The listing builds one solid part. Answer for the finished solid, in the listing's coordinates (mm). Face numbers are marked on the shaded views. A direction names the side the tool comes from. Give positions to 0.01 mm unless a question says otherwise; leave off trailing zeros. Write each loop counter-clockwise with the first axis right and the second up, starting at its lowest first coordinate (ties: lowest second). Pieces come first, ordered by that corner, then holes. Notation, with made-up numbers: (61.5, -7) -> (77.5, -7) arc R13 ccw to (77.5, 11) -> close; hole circle Ø10 at (14, 71). An arc over 180 degrees is marked (long way). Put each result on its own line as item: value. Start each with the question number.
1) Find the intervals of material crossed by line 1 along X through (y, z) = (-6.25, 0); line 2 along Y through (x, z) = (2.5, -3); line 3 along X through (y, z) = (-4, 0), in increasing order. Write a range as from..to.
2) Flat-ended cylindrical pins translate along their axes: pin 1 Ø10 at (y, z) = (1.5, -15.5) entering from -X; pin 2 Ø2 at (x, z) = (0, 12.5) entering from +Y; pin 3 Ø12 at (y, z) = (-61.5, 10) entering from +X. Find the tip coordinate at first contact, or state that the pin passes through.
3) For the marked faces 1, 2 and 3, determine the directions among +Z, -Z, +X, -X, +Y, -Y from which every point of the face is accessible in a straight line to the end or side of a thin tool.
4) A cutting plane is placed at B-B (y = -66). Write down the section's boundary in (x, z).
5) A cutting plane is placed at C-C (y = -46). Write down the section's boundary in (x, z), then the cut area to 3 significant figures.
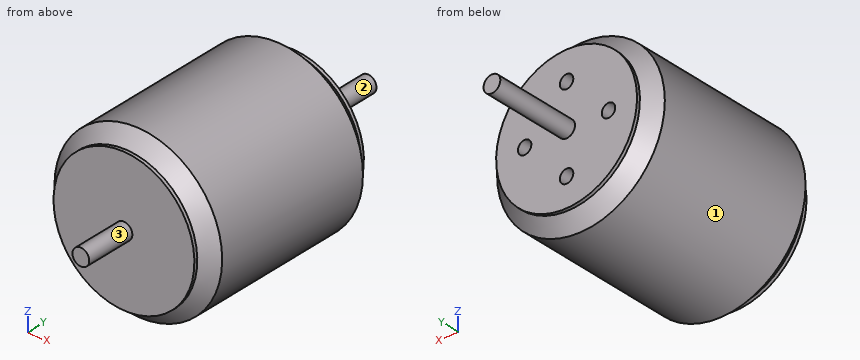
from build123d import *

# Parameters (mm, degrees)
SKETCH1_R           = 21
BOSS_EXTRUDE1_DEPTH = 59
SKETCH1_3_R         = 2.5
BOSS_EXTRUDE2_DEPTH = 26
SKETCH1_4_R         = 2
CUT_EXTRUDE1_DEPTH  = 10
BOSS_EXTRUDE3_START = -5
SKETCH1_5_R         = 25
SKETCH1_5_R_2       = 21
BOSS_EXTRUDE3_DEPTH = 49
CHAMFER1_SIZE       = 4
BOSS_EXTRUDE4_START = -74
SKETCH1_6_R         = 2.5
BOSS_EXTRUDE4_DEPTH = 15


with BuildPart() as part:
    # Sketch1 → Boss-Extrude1 (new body)
    with BuildSketch(Plane(origin=(0, 0, 0), x_dir=(1, 0, 0), z_dir=(0, 1, 0))):
        with Locations(Location((0, 0, 0), (0, 0, 270))):
            Circle(SKETCH1_R)
    extrude(amount=-BOSS_EXTRUDE1_DEPTH)

    # Sketch1<3> → Boss-Extrude2 (add)
    with BuildSketch(Plane(origin=(0, 0, 0), x_dir=(1, 0, 0), z_dir=(0, 1, 0))):
        with Locations(Location((0, 0, 0), (0, 0, 90))):
            Circle(SKETCH1_3_R)
    extrude(amount=BOSS_EXTRUDE2_DEPTH)

    # Sketch1<4> → Cut-Extrude1 (cut)
    with BuildSketch(Plane(origin=(0, 0, 0), x_dir=(1, 0, 0), z_dir=(0, 1, 0))):
        with Locations(Location((-12.5, 0, 0), (0, 0, 270))):
            Circle(SKETCH1_4_R)
        with Locations(Location((0, 12.5, 0), (0, 0, 270))):
            Circle(SKETCH1_4_R)
        with Locations(Location((12.5, 0, 0), (0, 0, 270))):
            Circle(SKETCH1_4_R)
        with Locations(Location((0, -12.5, 0), (0, 0, 270))):
            Circle(SKETCH1_4_R)
    extrude(amount=-CUT_EXTRUDE1_DEPTH, mode=Mode.SUBTRACT)

    # Sketch1<5> → Boss-Extrude3 (add)
    with BuildSketch(Plane(origin=(0, 0, 0), x_dir=(1, 0, 0), z_dir=(0, 1, 0)).offset(BOSS_EXTRUDE3_START)):
        with Locations(Location((0, 0, 0), (0, 0, 270))):
            Circle(SKETCH1_5_R)
        with Locations(Location((0, 0, 0), (0, 0, 270))):
            Circle(SKETCH1_5_R_2, mode=Mode.SUBTRACT)
    extrude(amount=-BOSS_EXTRUDE3_DEPTH)

    # Chamfer1
    chamfer1_edges = [part.edges().sort_by_distance(p)[0] for p in [
        (0, -5, -21),
        (0, -54, -21),
    ]]
    chamfer(chamfer1_edges, length=CHAMFER1_SIZE - 0.0001)  # a hair under: the kernel refuses the full size

    # Sketch1<6> → Boss-Extrude4 (add)
    with BuildSketch(Plane(origin=(0, 0, 0), x_dir=(1, 0, 0), z_dir=(0, 1, 0)).offset(BOSS_EXTRUDE4_START)):
        with Locations(Location((0, 0, 0), (0, 0, 90))):
            Circle(SKETCH1_6_R)
    extrude(amount=BOSS_EXTRUDE4_DEPTH)


solid = part.part
Reply:
1. line 1: x = -25..-14.5, -10.5..10.5, 14.5..25
1. line 2: y = -59..0
1. line 3: x = -24..-14.5, -10.5..10.5, 14.5..24
2. pin 1: stops at x = -18.77
2. pin 2: stops at y = -10
2. pin 3: stops at x = 21.73
3. face 1: +Y, -Y
3. face 2: +Y
3. face 3: -Y
4. outline: circle Ø5 at (0, 0)
5. outline: circle Ø50 at (0, 0)
5. area: 1,960 mm2
